from build123d import *

# Parameters (mm, degrees)
SKETCH_1_W          = 19.6
SKETCH_1_H          = 8.4
EXTRUDE_1_DEPTH     = 19.9
CHAMFER_1_SIZE      = 2
SKETCH_2_W          = 27.6
SKETCH_2_H          = 0.7
EXTRUDE_2_DEPTH     = 8.4
FILLET_1_R          = 3
CUT_EXTRUDE_1_REACH = 23.321
SKETCH_3_R          = 1.25
SKETCH_4_R          = 4.2
EXTRUDE_3_DEPTH     = 3.5
SKETCH_5_R          = 2
EXTRUDE_4_DEPTH     = 3


with BuildPart() as part:
    # 草圖1 → 填料-伸長1 (new body)
    with BuildSketch(Plane.XY):
        Rectangle(SKETCH_1_W, SKETCH_1_H)
    extrude(amount=EXTRUDE_1_DEPTH)

    # 導角1
    chamfer_1_edges = [part.edges().sort_by_distance(p)[0] for p in [
        (-9.8, 0, 19.9),
    ]]
    chamfer(chamfer_1_edges, length=CHAMFER_1_SIZE)

    # 草圖2 → 填料-伸長2 (add)
    with BuildSketch(Plane.XZ.offset(4.2)):
        with Locations((0, 15.35)):
            Rectangle(SKETCH_2_W, SKETCH_2_H)
    extrude(amount=-EXTRUDE_2_DEPTH)

    # 圓角1
    fillet_1_edges = [part.edges().sort_by_distance(p)[0] for p in [
        (13.8, -4.2, 15.35),
        (-13.8, -4.2, 15.35),
        (13.8, 4.2, 15.35),
        (-13.8, 4.2, 15.35),
    ]]
    fillet(fillet_1_edges, radius=FILLET_1_R)

    # 草圖3 → 除料-伸長1 (cut, up to next)
    with BuildSketch(Plane.XY.offset(15.7), mode=Mode.PRIVATE) as cut_extrude_1_sk1:
        with Locations((-11.75, 0)):
            Circle(SKETCH_3_R)
    cut_extrude_1_tool1 = extrude(cut_extrude_1_sk1.sketch, amount=-CUT_EXTRUDE_1_REACH, mode=Mode.PRIVATE) & part.part
    # 草圖3 → 除料-伸長1 (cut, up to next)
    with BuildSketch(Plane.XY.offset(15.7), mode=Mode.PRIVATE) as cut_extrude_1_sk2:
        with Locations((11.75, 0)):
            Circle(SKETCH_3_R)
    cut_extrude_1_tool2 = extrude(cut_extrude_1_sk2.sketch, amount=-CUT_EXTRUDE_1_REACH, mode=Mode.PRIVATE) & part.part
    add(cut_extrude_1_tool1.solids().sort_by_distance((-11.75, 0, 15.7))[0], mode=Mode.SUBTRACT)
    add(cut_extrude_1_tool2.solids().sort_by_distance((11.75, 0, 15.7))[0], mode=Mode.SUBTRACT)

    # 草圖4 → 填料-伸長3 (add)
    with BuildSketch(Plane.XY.offset(19.9)):
        with Locations((5.6, 0)):
            Circle(SKETCH_4_R)
    extrude(amount=EXTRUDE_3_DEPTH)

    # 草圖5 → 填料-伸長4 (add)
    with BuildSketch(Plane.XY.offset(23.4)):
        with Locations((5.6, 0)):
            Circle(SKETCH_5_R)
    extrude(amount=EXTRUDE_4_DEPTH)


solid = part.part
Build history of the part. All positions in model axes, mm. A direction names the side the tool comes from. Coordinates: 2 decimals unless noted, no trailing zeros. Order: outer loops, then holes, each group sorted by start corner. A loop starts at its lowest first (then second) coordinate and runs counter-clockwise, first axis right, second up. Notation, with made-up numbers: (-13, 64) -> (30, 64) arc R9 cw to (30, 81) -> close; hole circle Ø5 at (52.5, 84.25). An arc over 180 degrees is marked (long way). One line per item, written item: value.
(1) Slice it at C-C, the plane z = 6.25. List the corners of the cut face in (x, y), plus the area to 3 significant figures.
Checked values:
outline: (-9.8, -4.2) -> (9.8, -4.2) -> (9.8, 4.2) -> (-9.8, 4.2) -> close
area: 165 mm2
(2) Probe line 1 (X direction, y = 1, z = 15.5); line 2 (Z direction, x = 9.5, y = 2.5); line 3 (X direction, y = -3, z = 6.5). List the from-to ranges inside material, lowest first. Write a range as [from, to].
Checked values:
line 1: [-13.8, -12.5], [-11, 11], [12.5, 13.8]
line 2: [0, 19.9]
line 3: [-9.8, 9.8]
(3) Slice it at B-B, the plane y = -2.75. List the corners of the cut face in (x, z), plus the area to 3 significant figures.
Checked values:
outline: (-13.37, 15) -> (-9.8, 15) -> (-9.8, 0) -> (9.8, 0) -> (9.8, 15) -> (13.37, 15) -> (13.37, 15.7) -> (9.8, 15.7) -> (9.8, 19.9) -> (8.77, 19.9) -> (8.77, 23.4) -> (2.43, 23.4) -> (2.43, 19.9) -> (-7.8, 19.9) -> (-9.8, 17.9) -> (-9.8, 15.7) -> (-13.37, 15.7) -> close
area: 415 mm2
(4) Tool access for faces 1 (the flat face through (-10, 0, 15.7)), 2 (the flat face through (10, 0, 15.7)), 3 (the flat face through (9, -3, 19.9)): list every direction of +Z, -Z, +X, -X, +Y, -Y with a clear straight run to the whole face (end or side of a thin tool).
Checked values:
face 1: +Z, -X, +Y, -Y
face 2: +Z, +X, +Y, -Y
face 3: +Z, +X, -Y
(5) Drop flat-ended pins along their axis: pin 1 Ø1.2 at (x, y) = (12.5, -1.5) entering from +Z; pin 2 Ø4 at (y, z) = (-1.5, 23.5) entering from -X; pin 3 Ø1.2 at (x, y) = (11, -0.5) entering from -Z; pin 4 Ø2 at (x, y) = (-11.75, 0) entering from -Z. Give the stop position or say it passes through.
Checked values:
pin 1: z = 15.7
pin 2: x = 1.4
pin 3: z = 15
pin 4: through
(6) Slice it at A-A, the plane x = 11.75. List the corners of the cut face in (y, z), plus the area to 3 significant figures.
Checked values:
outline: (-4.05, 15) -> (-1.25, 15) -> (-1.25, 15.7) -> (-4.05, 15.7) -> close; (1.25, 15) -> (4.05, 15) -> (4.05, 15.7) -> (1.25, 15.7) -> close
area: 3.91 mm2
(7) Slice it at D-D, the plane x = 4. List the corners of the cut face in (y, z).
Checked values:
outline: (-4.2, 0) -> (4.2, 0) -> (4.2, 19.9) -> (3.88, 19.9) -> (3.88, 23.4) -> (1.2, 23.4) -> (1.2, 26.4) -> (-1.2, 26.4) -> (-1.2, 23.4) -> (-3.88, 23.4) -> (-3.88, 19.9) -> (-4.2, 19.9) -> close
